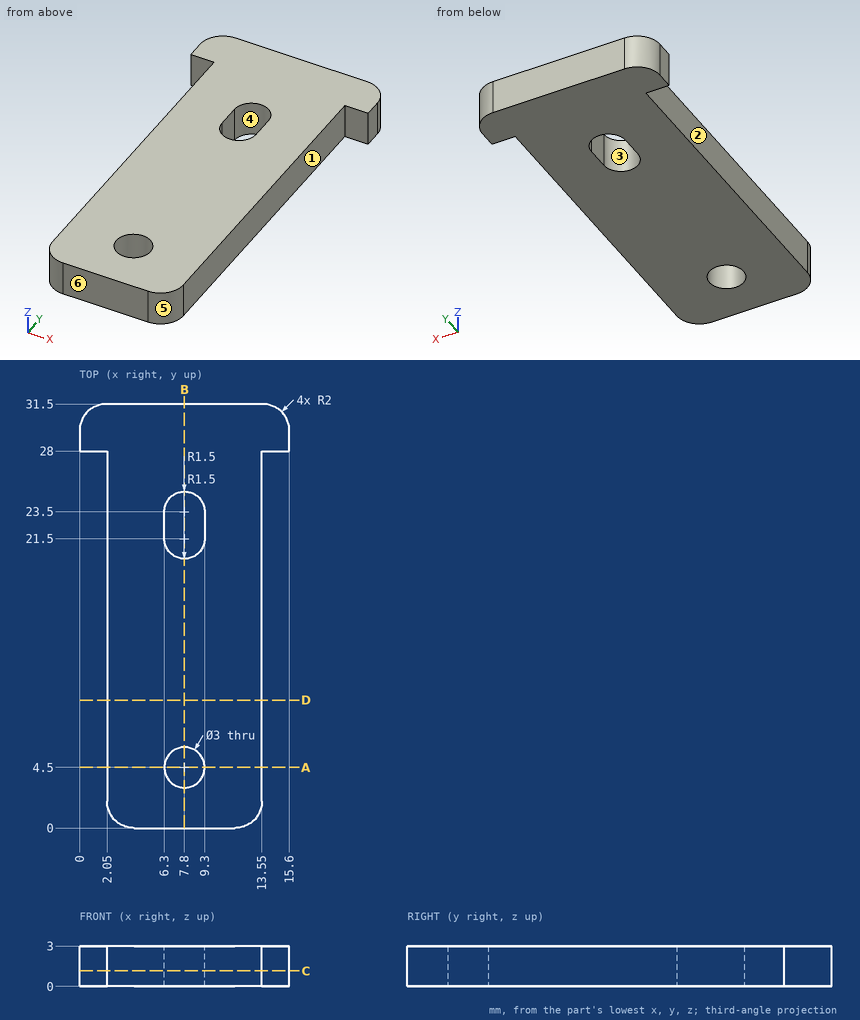
Study the drawing (mm; zero at the part's minimum x, y, z) and answer. A direction names the side the tool comes from. Coordinates: 2 decimals unless noted, no trailing zeros. Write each loop counter-clockwise with the first axis right and the second up, starting at its lowest first coordinate (ties: lowest second). Pieces come first, ordered by that corner, then holes. Notation, with made-up numbers: (-22.5, 53.25) - (9.5, 53.25) arc R9 ccw to (9.5, 65.25) - close; hole circle Ø9 at (-5, 56.25). An arc over 180 degrees is marked (long way). Return JSON: item names as keys, results as strings. Group by question number.
1. A cutting plane is placed at D-D, the plane y = 9.5. Determine the outline of the cut face in (x, z).
2. Straight lines are drawn through the part: L1, parallel to Y at x = 7.8, z = 1.95; L2, parallel to Y at x = 9, z = 2.3; L3, parallel to X at y = 22, z = 1.9. For each, find the intervals that lie inside material, in ascending order.
3. Given pin 1 (1 mm diameter, centred on y = 25.5, z = 2.5, fed in from +X); pin 2 (1.6 mm diameter, centred on x = 15, z = 1, fed in from -Y); pin 3 (4 mm diameter, centred on x = 12, y = 16.5, fed in from -Z); pin 4 (1.5 mm diameter, centred on y = 20.5, z = 1, fed in from -X), each flat-ended and moving along its own axis, determine where each tip first touches the part or whether it passes through.
4. Determine the mould class of the marked faces 4, 5 and 6 for opening direction X: released by +X, released by -X, zero draft, split by the parting line, or undercut.
5. Which of the six approach directions +Z, -Z, +X, -X, +Y, -Y give full straight-line access (tool end or side, diameter ignored) to the marked faces 1, 2 and 3?
6. A cutting plane is placed at C-C, the plane z = 1.15. Determine the outline of the cut face in (x, y), plus the area to 3 significant figures.
7. A cutting plane is placed at A-A, the plane y = 4.5. Determine the outline of the cut face in (x, z).
8. A cutting plane is placed at B-B, the plane x = 7.8. Determine the outline of the cut face in (y, z).
Ans:
{
 "1": {"outline": "(2.05, 0) - (13.55, 0) - (13.55, 3) - (2.05, 3) - close"},
 "2": {"L1": "0 to 3, 6 to 20, 25 to 31.5", "L2": "0 to 3.6, 5.4 to 20.6, 24.4 to 31.5", "L3": "2.05 to 6.3, 9.3 to 13.55"},
 "3": {"pin 1": "x = 13.55", "pin 2": "y = 28", "pin 3": "z = 0", "pin 4": "x = 2.05"},
 "4": {"face 4": "undercut", "face 5": "released by +X", "face 6": "zero draft"},
 "5": {"face 1": "+Z, -Z, +X, -Y", "face 2": "+Z, -Z, -X, -Y", "face 3": "+Z, -Z"},
 "6": {"outline": "(0, 28) - (2.05, 28) - (2.05, 2) arc R2 ccw to (4.05, 0) - (11.55, 0) arc R2 ccw to (13.55, 2) - (13.55, 28) - (15.6, 28) - (15.6, 29.5) arc R2 ccw to (13.6, 31.5) - (2, 31.5) arc R2 ccw to (0, 29.5) - close; hole circle Ø3 at (7.8, 4.5); hole (6.3, 21.5) arc R1.5 ccw to (9.3, 21.5) - (9.3, 23.5) arc R1.5 ccw to (6.3, 23.5) - close", "area": "353 mm²"},
 "7": {"outline": "(2.05, 0) - (6.3, 0) - (6.3, 3) - (2.05, 3) - close; (9.3, 0) - (13.55, 0) - (13.55, 3) - (9.3, 3) - close"},
 "8": {"outline": "(0, 0) - (3, 0) - (3, 3) - (0, 3) - close; (6, 0) - (20, 0) - (20, 3) - (6, 3) - close; (25, 0) - (31.5, 0) - (31.5, 3) - (25, 3) - close"}
}
